Verification items for the finished model (mm, model axes). A direction names the side the tool comes from. Give positions to 0.01 mm unless a question says otherwise; leave off trailing zeros. Loops run counter-clockwise (first coordinate to the right, second up) from the corner with the lowest first, then second, coordinate; pieces in that order, holes last. Notation, with made-up numbers: M 9.5,57 L 20.5,57 A12 ccw 20.5,63 Z; hole C 7,-25 d9. An arc over 180 degrees is marked long. Answer in a Markdown table with one row per item.
```python
from build123d import *

# Parameters (mm, degrees)
SKETCH3_R                = 2.15
BOSS_EXTRUDE1_DEPTH      = 40
BOSS_EXTRUDE1_DEPTH_BACK = 40


with BuildPart() as part:
    # Sketch3 → Boss-Extrude1 (new body, two sides)
    with BuildSketch(Plane.XY) as boss_extrude1_sk:
        with BuildLine():
            Line((3.2874, 10), (8, 10))
            ThreePointArc((8, 10), (9.414213562, 9.414213562), (10, 8))
            Line((10, 8), (10, 3.2874))
            ThreePointArc((10, 3.2874), (9.76937588, 2.73062412), (9.2126, 2.5))
            Line((9.2126, 2.5), (8.5048, 2.5))
            ThreePointArc((8.5048, 2.5), (8.289273853, 2.589273853), (8.2, 2.8048))
            Line((8.2, 2.8048), (8.2, 4.9118))
            ThreePointArc((8.2, 4.9118), (7.682565253, 5.686195824), (6.769103096, 5.504496904))
            Line((6.769103096, 5.504496904), (4.478679656, 3.214073464))
            ThreePointArc((4.478679656, 3.214073464), (3.828361402, 2.240803418), (3.6, 1.092753121))
            Line((3.6, 1.092753121), (3.6, -1.092753121))
            ThreePointArc((3.6, -1.092753121), (3.828361402, -2.240803418), (4.478679656, -3.214073464))
            Line((4.478679656, -3.214073464), (6.769103096, -5.504496904))
            ThreePointArc((6.769103096, -5.504496904), (7.682565253, -5.686195824), (8.2, -4.9118))
            Line((8.2, -4.9118), (8.2, -2.8048))
            ThreePointArc((8.2, -2.8048), (8.289273853, -2.589273853), (8.5048, -2.5))
            Line((8.5048, -2.5), (9.2126, -2.5))
            ThreePointArc((9.2126, -2.5), (9.76937588, -2.73062412), (10, -3.2874))
            Line((10, -3.2874), (10, -8))
            ThreePointArc((10, -8), (9.414213562, -9.414213562), (8, -10))
            Line((8, -10), (3.2874, -10))
            ThreePointArc((3.2874, -10), (2.73062412, -9.76937588), (2.5, -9.2126))
            Line((2.5, -9.2126), (2.5, -8.5048))
            ThreePointArc((2.5, -8.5048), (2.589273853, -8.289273853), (2.8048, -8.2))
            Line((2.8048, -8.2), (4.9118, -8.2))
            ThreePointArc((4.9118, -8.2), (5.686195824, -7.682565253), (5.504496904, -6.769103096))
            Line((5.504496904, -6.769103096), (3.214073464, -4.478679656))
            ThreePointArc((3.214073464, -4.478679656), (2.240803418, -3.828361402), (1.092753121, -3.6))
            Line((1.092753121, -3.6), (-1.092753121, -3.6))
            ThreePointArc((-1.092753121, -3.6), (-2.240803418, -3.828361402), (-3.214073464, -4.478679656))
            Line((-3.214073464, -4.478679656), (-5.504496904, -6.769103096))
            ThreePointArc((-5.504496904, -6.769103096), (-5.686195824, -7.682565253), (-4.9118, -8.2))
            Line((-4.9118, -8.2), (-2.8048, -8.2))
            ThreePointArc((-2.8048, -8.2), (-2.589273853, -8.289273853), (-2.5, -8.5048))
            Line((-2.5, -8.5048), (-2.5, -9.2126))
            ThreePointArc((-2.5, -9.2126), (-2.73062412, -9.76937588), (-3.2874, -10))
            Line((-3.2874, -10), (-8, -10))
            ThreePointArc((-8, -10), (-9.414213562, -9.414213562), (-10, -8))
            Line((-10, -8), (-10, -3.2874))
            ThreePointArc((-10, -3.2874), (-9.76937588, -2.73062412), (-9.2126, -2.5))
            Line((-9.2126, -2.5), (-8.5048, -2.5))
            ThreePointArc((-8.5048, -2.5), (-8.289273853, -2.589273853), (-8.2, -2.8048))
            Line((-8.2, -2.8048), (-8.2, -4.9118))
            ThreePointArc((-8.2, -4.9118), (-7.682565253, -5.686195824), (-6.769103096, -5.504496904))
            Line((-6.769103096, -5.504496904), (-4.478679656, -3.214073464))
            ThreePointArc((-4.478679656, -3.214073464), (-3.828361402, -2.240803418), (-3.6, -1.092753121))
            Line((-3.6, -1.092753121), (-3.6, 1.092753121))
            ThreePointArc((-3.6, 1.092753121), (-3.828361402, 2.240803418), (-4.478679656, 3.214073464))
            Line((-4.478679656, 3.214073464), (-6.769103096, 5.504496904))
            ThreePointArc((-6.769103096, 5.504496904), (-7.682565253, 5.686195824), (-8.2, 4.9118))
            Line((-8.2, 4.9118), (-8.2, 2.8048))
            ThreePointArc((-8.2, 2.8048), (-8.289273853, 2.589273853), (-8.5048, 2.5))
            Line((-8.5048, 2.5), (-9.2126, 2.5))
            ThreePointArc((-9.2126, 2.5), (-9.76937588, 2.73062412), (-10, 3.2874))
            Line((-10, 3.2874), (-10, 8))
            ThreePointArc((-10, 8), (-9.414213562, 9.414213562), (-8, 10))
            Line((-8, 10), (-3.2874, 10))
            ThreePointArc((-3.2874, 10), (-2.73062412, 9.76937588), (-2.5, 9.2126))
            Line((-2.5, 9.2126), (-2.5, 8.5048))
            ThreePointArc((-2.5, 8.5048), (-2.589273853, 8.289273853), (-2.8048, 8.2))
            Line((-2.8048, 8.2), (-4.9118, 8.2))
            ThreePointArc((-4.9118, 8.2), (-5.686195824, 7.682565253), (-5.504496904, 6.769103096))
            Line((-5.504496904, 6.769103096), (-3.214073464, 4.478679656))
            ThreePointArc((-3.214073464, 4.478679656), (-2.240803418, 3.828361402), (-1.092753121, 3.6))
            Line((-1.092753121, 3.6), (1.092753121, 3.6))
            ThreePointArc((1.092753121, 3.6), (2.240803418, 3.828361402), (3.214073464, 4.478679656))
            Line((3.214073464, 4.478679656), (5.504496904, 6.769103096))
            ThreePointArc((5.504496904, 6.769103096), (5.686195824, 7.682565253), (4.9118, 8.2))
            Line((4.9118, 8.2), (2.8048, 8.2))
            ThreePointArc((2.8048, 8.2), (2.589273853, 8.289273853), (2.5, 8.5048))
            Line((2.5, 8.5048), (2.5, 9.2126))
            ThreePointArc((2.5, 9.2126), (2.73062412, 9.76937588), (3.2874, 10))
        make_face()
        Circle(SKETCH3_R, mode=Mode.SUBTRACT)
    extrude(amount=BOSS_EXTRUDE1_DEPTH)
    extrude(boss_extrude1_sk.sketch, amount=-BOSS_EXTRUDE1_DEPTH_BACK)


solid = part.part
```
Item 1: Release check for a two-part mould opening along X. For faces 1 (the flat face through (-6, 10, 1)), 2 (the flat face through (10, 6, 1)), 3 (the cylindrical face through (-7.7, -5.68, 0.56)) record: released by +X, released by -X, zero draft, split by the parting line, or undercut.
Reported:
| item | result |
|---|---|
| face 1 | zero draft |
| face 2 | released by +X |
| face 3 | undercut |
Item 2: Go/stop test with flat-tipped pins: pin 1 (4 mm diameter, centred on x = -7.5, y = 0, fed in from +Z); pin 2 (0.7 mm diameter, centred on y = -0.5, z = -2, fed in from +X); pin 3 (1 mm diameter, centred on y = -0.5, z = -19, fed in from -X); pin 4 (3 mm diameter, centred on x = -2, z = -21, fed in from +Y). Record where each tip stops, or that it passes through.
Reported:
| item | result |
|---|---|
| pin 1 | passes through |
| pin 2 | stops at x = 3.6 |
| pin 3 | stops at x = -3.6 |
| pin 4 | stops at y = 10 |
Item 3: Scan lines: L1, parallel to X at y = 5, z = -33.5; L2, parallel to X at y = 5.25, z = 24; L3, parallel to Y at x = 0, z = -21.5. Record each from-to range of solid material in increasing order. Write a range as [from, to].
Reported:
| item | result |
|---|---|
| L1 | x = [-10, -8.2], [-6.26, -3.74], [3.74, 6.26], [8.2, 10] |
| L2 | x = [-10, -8.13], [-6.51, -3.99], [3.99, 6.51], [8.13, 10] |
| L3 | y = [-3.6, -2.15], [2.15, 3.6] |
Item 4: Sectioned sample at A-A (x = 0). Record the cut outline in (y, z).
Reported:
| item | result |
|---|---|
| outline | M -3.6,-40 L -2.15,-40 L -2.15,40 L -3.6,40 Z; M 2.15,-40 L 3.6,-40 L 3.6,40 L 2.15,40 Z |
Item 5: Tool access check on faces 4 (the flat face through (0, -3.6, 1)), 5 (the flat face through (3.6, 0, 1)), 6 (the flat face through (6, -10, 1)), 7 (the flat face through (8.2, -4, 1)). Record the directions out of +Z, -Z, +X, -X, +Y, -Y that give a thin tool (end or side, any length) a straight path to the whole face; none if there is none.
Reported:
| item | result |
|---|---|
| face 4 | +Z, -Z, -Y |
| face 5 | +Z, -Z, +X |
| face 6 | +Z, -Z, +X, -X, -Y |
| face 7 | +Z, -Z |
